from build123d import *

# Parameters (mm, degrees)
CHAMFER_1_SIZE      = 0.5
SKETCH_2_R          = 1.5
CUT_EXTRUDE_1_DEPTH = 5
SKETCH_3_R          = 1
SKETCH_3_R_2        = 1.25
CUT_EXTRUDE_2_DEPTH = 5


with BuildPart() as part:
    # 草图1 → 旋转1 (revolve)
    with BuildSketch(Plane(origin=(0, 0, 0), x_dir=(1, 0, 0), z_dir=(0, 1, 0)), mode=Mode.PRIVATE) as revolve_1_sk:
        Polygon((0, 19), (1, 19), (1, 20), (3, 20), (3, 19), (4, 19), (4, 8.5), (5, 8.5), (5, 0), (0, 0), (-15, 0), (-15, 15), (-14.5, 15), (-14.5, 20), (0, 20), align=None)
    revolve(revolve_1_sk.sketch.rotate(Axis((-9.646406884, 0, 0), (1, 0, 0)), 180), axis=Axis((-9.646406884, 0, 0), (1, 0, 0)))

    # 倒角1
    chamfer_1_edges = [part.edges().sort_by_distance(p)[0] for p in [
        (-14.5, 0, -15),
    ]]
    chamfer(chamfer_1_edges, length=CHAMFER_1_SIZE - 0.0001)  # a hair under: the kernel refuses the full size

    # 草图2 → 切除-拉伸1 (cut)
    with BuildSketch(Plane.ZY.offset(15)):
        with Locations((0, 10)):
            Circle(SKETCH_2_R)
        with Locations((10, 0)):
            Circle(SKETCH_2_R)
        with Locations((0, -10)):
            Circle(SKETCH_2_R)
        with Locations((-10, 0)):
            Circle(SKETCH_2_R)
    extrude(amount=-CUT_EXTRUDE_1_DEPTH, mode=Mode.SUBTRACT)

    # 草图3 → 切除-拉伸2 (cut)
    with BuildSketch(Plane(origin=(5, 0, 0), x_dir=(0, 0, -1), z_dir=(1, 0, 0))):
        with Locations((-8, 10.25)):
            Circle(SKETCH_3_R)
        with Locations(Location((8, 10.25, 0), (0, 0, 180))):
            Circle(SKETCH_3_R)
        with Locations((8, -10.25)):
            Circle(SKETCH_3_R)
        with Locations(Location((-8, -10.25, 0), (0, 0, 180))):
            Circle(SKETCH_3_R)
        with Locations((-11.844038585, 11.844038585)):
            Circle(SKETCH_3_R_2)
        with Locations((11.844038585, 11.844038585)):
            Circle(SKETCH_3_R_2)
        with Locations((11.844038585, -11.844038585)):
            Circle(SKETCH_3_R_2)
        with Locations((-11.844038585, -11.844038585)):
            Circle(SKETCH_3_R_2)
    extrude(amount=-CUT_EXTRUDE_2_DEPTH, mode=Mode.SUBTRACT)


solid = part.part
Verification items for the finished model (mm, model axes). A direction names the side the tool comes from. Coordinates: 2 decimals unless noted, no trailing zeros. Order: outer loops, then holes, each group sorted by start corner. A loop starts at its lowest first (then second) coordinate and runs counter-clockwise, first axis right, second up.
Item 1: Section check C-C, the plane x = -1. Enter the section's corners in (y, z).
Filled in:
outline: circle Ø40 at (0, 0)
Item 2: Material ranges on L1, parallel to X at y = 16, z = 10.5; L2, parallel to Y at x = 1.1, z = -8; L3, parallel to Z at x = 1.5, y = 12, recorded low to high.
Filled in:
L1: x = -14.5 to 0, 1 to 3
L2: y = -18.33 to -11.25, -9.25 to 9.25, 11.25 to 18.33
L3: z = -16 to -13.08, -10.6 to 10.6, 13.08 to 16
Item 3: Access from +Z, -Z, +X, -X, +Y, -Y to the whole of each face (thin tool, end or side, straight path). Record for faces 4 (the face through (1, 7, -18)), 5 (the face through (-12.535, 8.536, -0.325)), 6 (the face through (0, -10, 8)).
Filled in:
face 4: none
face 5: -X
face 6: +X
Item 4: Section check A-A, the plane x = -10.5. Enter the section's corners in (y, z).
Filled in:
outline: circle Ø40 at (0, 0); hole circle Ø3 at (-10, 0); hole circle Ø3 at (0, -10); hole circle Ø3 at (0, 10); hole circle Ø3 at (10, 0)
Item 5: Release check for a two-part mould opening along X. For faces 1 (the face through (2.028, 10.624, -11.573)), 2 (the face through (0, 7, 18)), 3 (the face through (-10, -10, 0)) record: +X half, -X half, draft (parallel to the pull), parting line (faces both ways), or undercut.
Filled in:
face 1: draft
face 2: undercut
face 3: -X half
Item 6: Depth check by flat-ended pin: pin 1 (10 mm diameter, centred on x = -2.5, z = 2.5, fed in from +Y); pin 2 (5 mm diameter, centred on y = 2.5, z = -13.5, fed in from +X); pin 3 (12 mm diameter, centred on x = 3, y = -7.5, fed in from -Z); pin 4 (10 mm diameter, centred on y = 16, z = 11.5, fed in from -X). Enter the tip coordinate at first touch or a pass-through.
Filled in:
pin 1: stops at y = 20
pin 2: stops at x = 4
pin 3: stops at z = -19.94
pin 4: stops at x = -15
